Source: three-view drawing plus pictorial views. Frame: mm from the lowest corner of the part. A direction names the side the tool comes from. Coordinates: 2 decimals unless noted, no trailing zeros. Loops run counter-clockwise (first coordinate to the right, second up) from the corner with the lowest first, then second, coordinate; pieces in that order, holes last. Notation, with made-up numbers: M -15.5,38 L 32.5,38 A21 ccw 32.5,53 Z; hole C 6,-39.75 d1. An arc over 180 degrees is marked long. Use a Markdown table: item, result. Add a question column.
1. Section A-A on z = 18. Output: boundary loops of the cut face in (x, y).
2. Section D-D on x = 3.75. Output: boundary loops of the cut face in (y, z), then the cut area to 3 significant figures.
3. Section B-B on x = 23.5. Output: boundary loops of the cut face in (y, z).
4. Set-up query: the marked faces 1 and 2. Return all of +Z, -Z, +X, -X, +Y, -Y with unobstructed straight access to the full face (end or side cutting, diameter ignored); none if empty.
5. Line query: L1, parallel to Y at x = 43.25, z = 0.45; L2, parallel to Z at x = 14, y = 22. Output: solid intervals per line, ascending. Write a range as [from, to].
6. Pin query (flat end, axial travel): pin 1 (12 mm diameter, centred on x = 7.5, y = 44, fed in from +Z); pin 2 (1.1 mm diameter, centred on y = 0.5, z = 20.5, fed in from +X); pin 3 (3 mm diameter, centred on x = 24.5, z = 6, fed in from +Y). Return the tip coordinate at first contact, or that it passes through.
7. Section C-C on y = 45.55. Output: boundary loops of the cut face in (x, z).
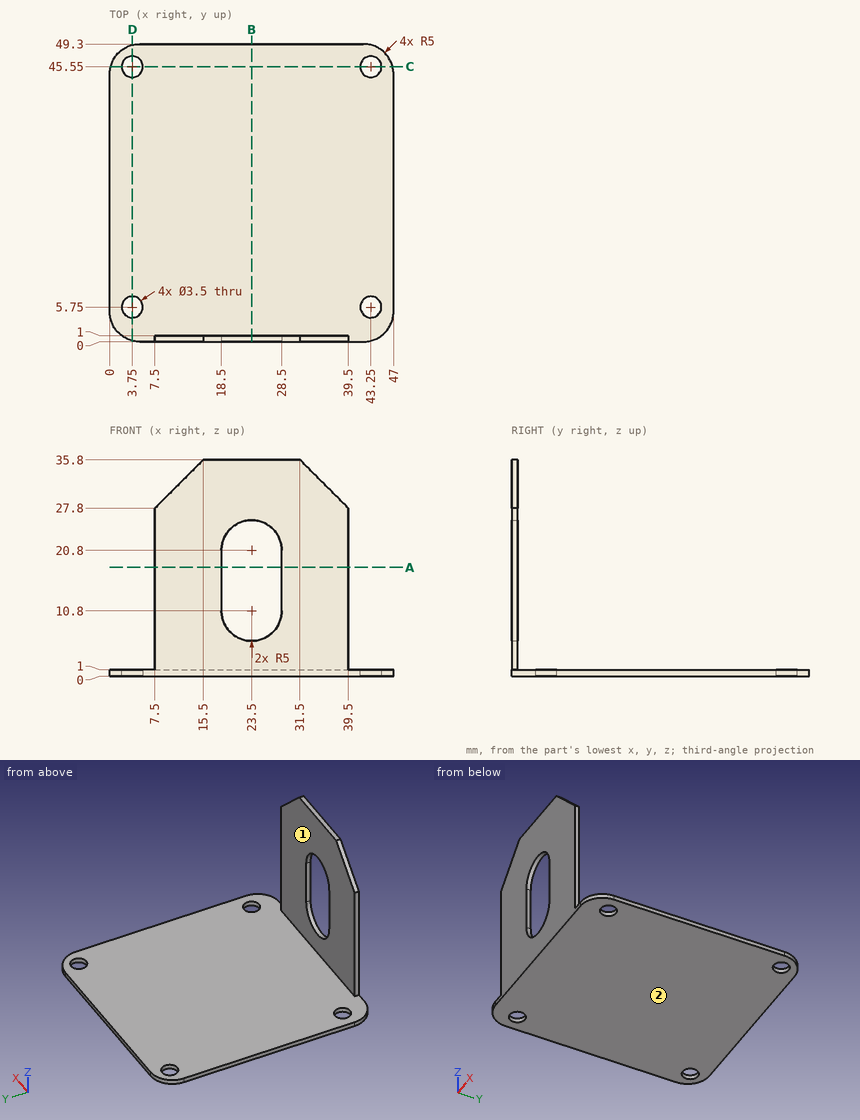
Answers below:
| question | item | result |
|---|---|---|
| 1 | outline | M 7.5,0 L 18.5,0 L 18.5,1 L 7.5,1 Z; M 28.5,0 L 39.5,0 L 39.5,1 L 28.5,1 Z |
| 2 | outline | M 0.16,0 L 4,0 L 4,1 L 0.16,1 Z; M 7.5,0 L 43.8,0 L 43.8,1 L 7.5,1 Z; M 47.3,0 L 49.14,0 L 49.14,1 L 47.3,1 Z |
| 2 | area | 42.0 mm² |
| 3 | outline | M 0,0 L 49.3,0 L 49.3,1 L 1,1 L 1,5.8 L 0,5.8 Z; M 0,25.8 L 1,25.8 L 1,35.8 L 0,35.8 Z |
| 4 | face 1 | +Z, +X, -X, +Y |
| 4 | face 2 | -Z, +X, -X, +Y, -Y |
| 5 | L1 | y = [0.16, 4], [7.5, 43.8], [47.3, 49.14] |
| 5 | L2 | z = [0, 1] |
| 6 | pin 1 | stops at z = 1 |
| 6 | pin 2 | stops at x = 39.5 |
| 6 | pin 3 | stops at y = 1 |
| 7 | outline | M 0.16,0 L 2,0 L 2,1 L 0.16,1 Z; M 5.5,0 L 41.5,0 L 41.5,1 L 5.5,1 Z; M 45,0 L 46.84,0 L 46.84,1 L 45,1 Z |
